Input: part model. Units: mm. Frame: model coordinates. A direction names the side the tool comes from. Give positions to 0.01 mm unless a question says otherwise; leave off trailing zeros. Write each loop counter-clockwise with the first axis right and the second up, starting at its lowest first coordinate (ties: lowest second). Pieces come first, ordered by that corner, then holes. Notation, with made-up numbers: (32.5, 26.25) - (51.5, 26.25) arc R10 ccw to (51.5, 32.25) - close; hole circle Ø1 at (-19, 75). An arc over 180 degrees is marked (long way). Use a Markdown table: item, result. Add a question column.
1. Pin query (flat end, axial travel): pin 1 (8 mm diameter, centred on x = 26.04, z = -26.04, fed in from +Y); pin 2 (1.9 mm diameter, centred on y = 2.5, z = 2.5, fed in from +X); pin 3 (3 mm diameter, centred on x = 7.5, y = 3, fed in from -Z). Return the tip coordinate at first contact, or that it passes through.
2. Material intervals for probe 1 along X at (y, z) = (13.5, -19.5); probe 2 along Z at (x, y) = (-54, 27.5); probe 3 along X at (y, z) = (28, -29), sorted ascending.
3. Set-up query: faces 4 (the cylindrical face through (29.49, 3.1, 29.65)), 5 (the conical face through (-31.754, 33.95, 30.384)), 6 (the cylindrical face through (23.375, 0.986, 24.652)). Return all of +Z, -Z, +X, -X, +Y, -Y with unobstructed straight access to the full face (end or side cutting, diameter ignored); none if empty.
4. Section query B-B, the plane y = 12. Count the separate pieces of the cut face and the enclosed holes in it, plus the area to 3 significant figures.
5. Mould query, pull axis Z, two halves, no side actions, for faces 1 (the conical face through (30.42, 7.84, -30.36)), 2 (the conical face through (-98.9, 0.2, -28.76)), 3 (the conical face through (-98.76, 0.2, 28.9)). Classes: released by +Z, released by -Z, zero draft, split by the parting line, or undercut.
6. Section query A-A, the plane x = -82. Return loops of the section in (y, z), plus the area to 3 significant figures.
```python
from build123d import *

# Parameters (mm, degrees)
BOSS_EXTRUDE4_DEPTH = 5
SKETCH6_W           = 70
SKETCH6_H           = 70
BOSS_EXTRUDE5_DEPTH = 30
SKETCH8_R           = 3
CUT_EXTRUDE1_DEPTH  = 2
FILLET1_R           = 7.5
SKETCH13_W          = 33.08628573
SKETCH13_H          = 65
CUT_EXTRUDE2_DEPTH  = 27.5
FILLET2_R           = 7.5
CHAMFER1_SIZE       = 1.25
CHAMFER2_SIZE       = 1.25


with BuildPart() as part:
    # Sketch5 → Boss-Extrude4 (new body)
    with BuildSketch(Plane(origin=(0, 0, 0), x_dir=(1, 0, 0), z_dir=(0, 1, 0))):
        with BuildLine():
            Line((-22.5, -32.5), (22.5, -32.5))
            ThreePointArc((22.5, -32.5), (29.571067812, -29.571067812), (32.5, -22.5))
            Line((32.5, -22.5), (32.5, 22.5))
            ThreePointArc((32.5, 22.5), (29.571067812, 29.571067812), (22.5, 32.5))
            Line((22.5, 32.5), (-22.5, 32.5))
            ThreePointArc((-22.5, 32.5), (-29.571067812, 29.571067812), (-32.5, 22.5))
            Line((-32.5, 22.5), (-32.5, -22.5))
            ThreePointArc((-32.5, -22.5), (-29.571067812, -29.571067812), (-22.5, -32.5))
        make_face()
    extrude(amount=BOSS_EXTRUDE4_DEPTH)

    # Sketch6 → Boss-Extrude5 (add)
    with BuildSketch(Plane(origin=(0, 5, 0), x_dir=(1, 0, 0), z_dir=(0, 1, 0))):
        Rectangle(SKETCH6_W, SKETCH6_H)
    extrude(amount=BOSS_EXTRUDE5_DEPTH)

    # Sketch8 → Cut-Extrude1 (cut)
    with BuildSketch(Plane.XZ):
        with Locations(Location((26.037533906, -26.035533906, 0), (0, 0, 270))):
            Circle(SKETCH8_R)
        with Locations(Location((26.036533906, 26.036533906, 0), (0, 0, 270))):
            Circle(SKETCH8_R)
        with BuildLine():
            ThreePointArc((-23.035533906, 26.035533906), (-24.887483609, 28.807172503), (-28.156854249, 28.156854249))
            Line((-28.156854249, 28.156854249), (-23.914213562, 23.914213562))
            ThreePointArc((-23.914213562, 23.914213562), (-23.263895308, 24.887483609), (-23.035533906, 26.035533906))
        make_face()
        with BuildLine():
            Line((-23.914213562, 23.914213562), (-28.156854249, 28.156854249))
            ThreePointArc((-28.156854249, 28.156854249), (-28.156854249, 23.914213562), (-23.914213562, 23.914213562))
        make_face()
        with Locations(Location((-26.034533906, -26.036533906, 0), (0, 0, 270))):
            Circle(SKETCH8_R)
    extrude(amount=-CUT_EXTRUDE1_DEPTH, mode=Mode.SUBTRACT)

    # Mirror1: part across plane


with BuildPart() as part_1:
    add(part.part)
    add(part.part.mirror(Plane(origin=(-35, 35, -35), x_dir=(0, 0, 1), z_dir=(1, 0, 0))))

    # Fillet1
    fillet1_edges = [part_1.edges().sort_by_distance(p)[0] for p in [
        (35, 20, 35),
        (35, 20, -35),
        (-105, 20, 35),
        (-105, 20, -35),
    ]]
    fillet(fillet1_edges, radius=FILLET1_R)

    # Sketch13 → Cut-Extrude2 (cut)
    with BuildSketch(Plane(origin=(0, 35, 0), x_dir=(1, 0, 0), z_dir=(0, 1, 0))):
        with BuildLine():
            Line((-97.5, -32.5), (-71.83628573, -32.5))
            Line((-71.83628573, -32.5), (-71.83628573, 32.5))
            Line((-71.83628573, 32.5), (-97.5, 32.5))
            ThreePointArc((-97.5, 32.5), (-101.035533906, 31.035533906), (-102.5, 27.5))
            Line((-102.5, 27.5), (-102.5, -27.5))
            ThreePointArc((-102.5, -27.5), (-101.035533906, -31.035533906), (-97.5, -32.5))
        make_face()
        with Locations((-52.793142865, 0)):
            Rectangle(SKETCH13_W, SKETCH13_H)
        with Locations((-17.206857135, 0)):
            Rectangle(SKETCH13_W, SKETCH13_H)
        with BuildLine():
            Line((1.83628573, 32.5), (1.83628573, -32.5))
            Line((1.83628573, -32.5), (27.5, -32.5))
            ThreePointArc((27.5, -32.5), (31.035533906, -31.035533906), (32.5, -27.5))
            Line((32.5, -27.5), (32.5, 27.5))
            ThreePointArc((32.5, 27.5), (31.035533906, 31.035533906), (27.5, 32.5))
            Line((27.5, 32.5), (1.83628573, 32.5))
        make_face()
    extrude(amount=-CUT_EXTRUDE2_DEPTH, mode=Mode.SUBTRACT)

    # Fillet2
    fillet2_edges = [part_1.edges().sort_by_distance(p)[0] for p in [
        (-71.83628573, 21.25, -32.5),
        (-71.83628573, 21.25, 32.5),
        (-36.25, 21.25, -32.5),
        (-36.25, 21.25, 32.5),
        (-69.33628573, 21.25, 32.5),
        (-69.33628573, 21.25, -32.5),
        (-0.66371427, 21.25, -32.5),
        (-0.66371427, 21.25, 32.5),
        (-33.75, 21.25, 32.5),
        (-33.75, 21.25, -32.5),
        (1.83628573, 21.25, 32.5),
        (1.83628573, 21.25, -32.5),
    ]]
    fillet(fillet2_edges, radius=FILLET2_R)

    # Chamfer1
    chamfer1_edges = [part_1.edges().sort_by_distance(p)[0] for p in [
        (-88.418142865, 7.5, 32.5),
        (-101.035533906, 7.5, 31.035533906),
        (-102.5, 7.5, 0),
        (-101.035533906, 7.5, -31.035533906),
        (-101.035533906, 35, -31.035533906),
        (-102.5, 35, 0),
        (-101.035533906, 35, 31.035533906),
        (-88.418142865, 35, 32.5),
        (18.418142865, 7.5, -32.5),
        (31.035533906, 7.5, -31.035533906),
        (32.5, 7.5, 0),
        (31.035533906, 7.5, 31.035533906),
        (31.035533906, 35, 31.035533906),
        (32.5, 35, 0),
        (31.035533906, 35, -31.035533906),
        (18.418142865, 35, -32.5),
        (-71.83628573, 35, 0),
        (-71.83628573, 7.5, 0),
        (-88.418142865, 7.5, -32.5),
        (-74.032984871, 7.5, -30.303300859),
        (-74.032984871, 7.5, 30.303300859),
        (-36.25, 35, 0),
        (-36.25, 7.5, 0),
        (-52.793142865, 35, 32.5),
        (-52.793142865, 7.5, 32.5),
        (-52.793142865, 7.5, -32.5),
        (-69.33628573, 7.5, 0),
        (-38.446699141, 7.5, -30.303300859),
        (-67.139586589, 7.5, -30.303300859),
        (-67.139586589, 7.5, 30.303300859),
        (-38.446699141, 7.5, 30.303300859),
        (-0.66371427, 35, 0),
        (-0.66371427, 7.5, 0),
        (-17.206857135, 35, 32.5),
        (-17.206857135, 7.5, 32.5),
        (-17.206857135, 7.5, -32.5),
        (-33.75, 7.5, 0),
        (-2.860413411, 7.5, -30.303300859),
        (-31.553300859, 7.5, -30.303300859),
        (-31.553300859, 7.5, 30.303300859),
        (-2.860413411, 7.5, 30.303300859),
        (-69.33628573, 35, 0),
        (-33.75, 35, 0),
        (18.418142865, 35, 32.5),
        (18.418142865, 7.5, 32.5),
        (1.83628573, 35, 0),
        (1.83628573, 7.5, 0),
        (4.032984871, 7.5, -30.303300859),
        (4.032984871, 7.5, 30.303300859),
        (-17.206857135, 35, -32.5),
        (-52.793142865, 35, -32.5),
        (-88.418142865, 35, -32.5),
        (-74.032984871, 35, 30.303300859),
        (-38.446699141, 35, 30.303300859),
        (-2.860413411, 35, 30.303300859),
        (-67.139586589, 35, 30.303300859),
        (-31.553300859, 35, 30.303300859),
        (4.032984871, 35, 30.303300859),
        (4.032984871, 35, -30.303300859),
        (-31.553300859, 35, -30.303300859),
        (-67.139586589, 35, -30.303300859),
        (-2.860413411, 35, -30.303300859),
        (-38.446699141, 35, -30.303300859),
        (-74.032984871, 35, -30.303300859),
    ]]
    chamfer(chamfer1_edges, length=CHAMFER1_SIZE - 0.0001)  # a hair under: the kernel refuses the full size

    # Chamfer2
    chamfer2_edges = [part_1.edges().sort_by_distance(p)[0] for p in [
        (32.5, 0, 0),
        (-35, 5, -35),
        (29.571067812, 0, 29.571067812),
        (-35, 5, 35),
        (-105, 5, 0),
        (35, 5, 0),
        (-102.803300859, 5, -32.803300859),
        (0, 0, 32.5),
        (-102.803300859, 5, 32.803300859),
        (32.803300859, 5, 32.803300859),
        (32.803300859, 5, -32.803300859),
        (-29.571067812, 0, 29.571067812),
        (-40.428932188, 0, 29.571067812),
        (-70, 0, 32.5),
        (-99.571067812, 0, 29.571067812),
        (-102.5, 0, 0),
        (-99.571067812, 0, -29.571067812),
        (-70, 0, -32.5),
        (-40.428932188, 0, -29.571067812),
        (-37.5, 0, 0),
        (-32.5, 0, 0),
        (-29.571067812, 0, -29.571067812),
        (0, 0, -32.5),
        (29.571067812, 0, -29.571067812),
    ]]
    chamfer(chamfer2_edges, length=CHAMFER2_SIZE)


solid = part_1.part
```
Result sheet:
| question | item | result |
|---|---|---|
| 1 | pin 1 | stops at y = 7.5 |
| 1 | pin 2 | stops at x = 32.5 |
| 1 | pin 3 | stops at z = -32.5 |
| 2 | probe 1 | x = -105 to -102.5, -71.84 to -69.34, -36.25 to -33.75, -0.66 to 1.84, 32.5 to 35 |
| 2 | probe 2 | z = -35 to -32.5, 32.5 to 35 |
| 2 | probe 3 | x = -104.85 to -102.27, -72.99 to -68.18, -37.41 to -32.59, -1.82 to 2.99, 32.27 to 34.85 |
| 3 | face 4 | +Z, +X, -Y |
| 3 | face 5 | +Y |
| 3 | face 6 | -Y |
| 4 | separate pieces | 1 |
| 4 | enclosed holes | 4 |
| 4 | area | 1,630 mm² |
| 5 | face 1 | undercut |
| 5 | face 2 | released by -Z |
| 5 | face 3 | released by +Z |
| 6 | outline | (0, -31.25) - (1.25, -32.5) - (5, -32.5) - (5, -33.75) - (6.25, -35) - (35, -35) - (35, -33.75) - (33.75, -32.5) - (8.75, -32.5) - (7.5, -31.25) - (7.5, 31.25) - (8.75, 32.5) - (33.75, 32.5) - (35, 33.75) - (35, 35) - (6.25, 35) - (5, 33.75) - (5, 32.5) - (1.25, 32.5) - (0, 31.25) - close |
| 6 | area | 634 mm² |
